Check sheet for the modelled part. Datum: model origin and axes. Units: mm. A direction names the side the tool comes from. Round coordinates to 2 decimals unless told otherwise and drop trailing zeros. Loops run counter-clockwise (first coordinate to the right, second up) from the corner with the lowest first, then second, coordinate; pieces in that order, holes last. Notation, with made-up numbers: (10, 25.5) -> (53, 25.5) arc R14 cw to (53, 48.5) -> close; hole circle Ø1 at (-16.5, 59.5). An arc over 180 degrees is marked (long way). Return JSON: item names as keys, results as strings.
from build123d import *

# Parameters (mm, degrees)
F0_R           = 2.5
F0_R_2         = 2.3
F1_DEPTH       = 39.5
F4_D           = 2.5
F4_CSINK_D     = 4.5
F4_CSINK_ANGLE = 90
F5_START       = 4
F5_DEPTH       = 0.5
F7_START       = -4
F6_R           = 2.5
F6_R_2         = 2.3
F7_DEPTH       = 0.5
F8_SIZE        = 0.2
F9_SIZE        = 0.1


with BuildPart() as f1:
    # F0 (on Front) → F1 (new body)
    with BuildSketch(Plane.XZ):
        Circle(F0_R)
        Circle(F0_R_2, mode=Mode.SUBTRACT)
        Circle(F0_R_2)
    extrude(amount=F1_DEPTH)

    # F4 (through all)
    with Locations(Plane.XY.offset(3)):
        with Locations((0, -28)):
            CounterSinkHole(F4_D / 2, F4_CSINK_D / 2, counter_sink_angle=F4_CSINK_ANGLE)

    # F0 (on Front) → F5 (cut)
    with BuildSketch(Plane.XZ.offset(F5_START)):
        Circle(F0_R)
        Circle(F0_R_2, mode=Mode.SUBTRACT)
    extrude(amount=F5_DEPTH, mode=Mode.SUBTRACT)

    # F6 (on face) → F7 (cut)
    with BuildSketch(Plane.XZ.offset(39.5).offset(F7_START)):
        Circle(F6_R)
        Circle(F6_R_2, mode=Mode.SUBTRACT)
    extrude(amount=-F7_DEPTH, mode=Mode.SUBTRACT)

    # F8
    f8_edges = [f1.edges().sort_by_distance(p)[0] for p in [
        (-2.5, -39.5, 0),
        (-2.5, 0, 0),
    ]]
    chamfer(f8_edges, length=F8_SIZE)

    # F9
    f9_edges = [f1.edges().sort_by_distance(p)[0] for p in [
        (-2.5, -4, 0),
        (-2.5, -4.5, 0),
        (-2.5, -35, 0),
        (-2.5, -35.5, 0),
    ]]
    chamfer(f9_edges, length=F9_SIZE)


solid = f1.part
Q1. Draft check along X on faces 1 (the flat face through (0, 0, 0)), 2 (the cylindrical face through (-0.54, -37.42, -2.44)), 3 (the cylindrical face through (1.25, -27.95, -0.28)). Enter one of: released by +X, released by -X, zero draft, split by the parting line, or undercut.
Results list:
{"face 1": "zero draft", "face 2": "split by the parting line", "face 3": "undercut"}
Q2. Section check A-A (y = -28). Record the boundary of the cut face in (x, z).
Results list:
{"outline": "(-1.35, 2.1) arc R2.5 ccw to (-1.25, -2.17) -> (-1.25, 2) -> close; (1.25, -2.17) arc R2.5 ccw to (1.35, 2.1) -> (1.25, 2) -> close"}
Q3. Tool access check on faces 4 (the cylindrical face through (-1.825, -35.254, -1.4)), 5 (the cylindrical face through (-0.54, -2.02, -2.44)). Record the directions out of +Z, -Z, +X, -X, +Y, -Y that give a thin tool (end or side, any length) a straight path to the whole face; none if there is none.
Results list:
{"face 4": "none", "face 5": "+Y, -Y"}
Q4. Go/stop test with a flat-tipped pin: pin 1 (1.5 mm diameter, centred on x = 2, z = 1, fed in from +Y). Record where the tip stops, or that it passes through.
Results list:
{"pin 1": "y = 0"}
Q5. Material ranges on line 1 (Y direction, x = 0, z = 1.05); line 2 (X direction, y = -28, z = 0.2); line 3 (Y direction, x = -0.7, z = -0.7), recorded low to high.
Results list:
{"line 1": "-39.5 to -29.25, -26.75 to 0", "line 2": "-2.49 to -1.25, 1.25 to 2.49", "line 3": "-39.5 to -29.04, -26.96 to 0"}
Q6. Section check B-B (y = -3). Record the boundary of the cut face in (x, z).
Results list:
{"outline": "circle Ø5 at (0, 0)"}
